from build123d import *
from build123d.topology import SkipClean

# Parameters (mm, degrees)
SKETCH1_W           = 30
SKETCH1_H           = 60
SKETCH1_R           = 1.75
BOSS_EXTRUDE1_DEPTH = 15
SKETCH4_R           = 1.75
BOSS_EXTRUDE3_DEPTH = 30
SKETCH5_W           = 5
SKETCH5_H           = 10
SKETCH5_W_2         = 10
CUT_EXTRUDE1_DEPTH  = 69.738635424
SKETCH6_W           = 7.5
SKETCH6_H           = 15
BOSS_EXTRUDE4_DEPTH = 30
SKETCH7_W           = 30
SKETCH7_H           = 15
BOSS_EXTRUDE5_DEPTH = 10
BOSS_EXTRUDE6_START = 30
SKETCH8_W           = 30
SKETCH8_H           = 15
SKETCH8_R           = 1.75
BOSS_EXTRUDE6_DEPTH = 30


with BuildPart() as part:
    # Sketch1 → Boss-Extrude1 (new body)
    with BuildSketch(Plane.XY):
        with Locations((15, 30)):
            Rectangle(SKETCH1_W, SKETCH1_H)
        with Locations((15, 10)):
            Circle(SKETCH1_R, mode=Mode.SUBTRACT)
    extrude(amount=BOSS_EXTRUDE1_DEPTH)

    # Sketch4 → Boss-Extrude3 (add)
    with BuildSketch(Plane(origin=(30, 0, 0), x_dir=(0, 0, -1), z_dir=(1, 0, 0))):
        with BuildLine():
            Line((-15, 15), (-20, 15))
            ThreePointArc((-20, 15), (-25, 20), (-20, 25))
            Line((-20, 25), (-15, 25))
            Line((-15, 25), (-15, 15))
        make_face()
        with Locations((-20, 20)):
            Circle(SKETCH4_R, mode=Mode.SUBTRACT)
    extrude(amount=-BOSS_EXTRUDE3_DEPTH)

    # Sketch5 → Cut-Extrude1 (cut, through all)
    with BuildSketch(Plane.XY.offset(15)):
        with Locations((2.5, 20)):
            Rectangle(SKETCH5_W, SKETCH5_H)
        with Locations((15, 20)):
            Rectangle(SKETCH5_W_2, SKETCH5_H)
        with Locations((27.5, 20)):
            Rectangle(SKETCH5_W, SKETCH5_H)
    extrude(amount=CUT_EXTRUDE1_DEPTH, mode=Mode.SUBTRACT)

    # Sketch6 → Boss-Extrude4 (add)
    with BuildSketch(Plane.XY.offset(15)):
        with Locations((3.75, 7.5)):
            Rectangle(SKETCH6_W, SKETCH6_H)
        with Locations((26.25, 7.5)):
            Rectangle(SKETCH6_W, SKETCH6_H)
    extrude(amount=BOSS_EXTRUDE4_DEPTH)

    # Sketch7 → Boss-Extrude5 (add)
    with BuildSketch(Plane.XY.offset(45)):
        with Locations((15, 7.5)):
            Rectangle(SKETCH7_W, SKETCH7_H)
    extrude(amount=BOSS_EXTRUDE5_DEPTH)

    # Sketch8 → Boss-Extrude6 (add)
    with SkipClean():  # the faces are left unmerged after this step: merging them gives an invalid solid
        with BuildSketch(Plane(origin=(0, 0, 0), x_dir=(-1, 0, 0), z_dir=(0, 0, -1)).offset(BOSS_EXTRUDE6_START)):
            with Locations((-15, 7.5)):
                Rectangle(SKETCH8_W, SKETCH8_H)
            with Locations((-15, 10)):
                Circle(SKETCH8_R, mode=Mode.SUBTRACT)
        extrude(amount=-BOSS_EXTRUDE6_DEPTH)


solid = part.part
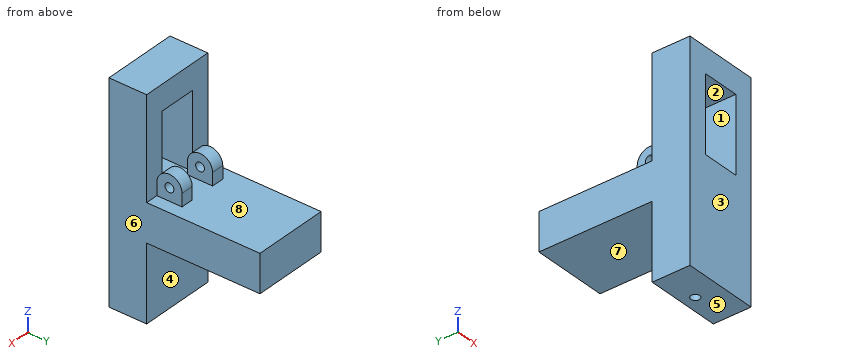
Geometry: final body of the model. Coordinates: model frame, mm. Face numbers are marked on the shaded views. A direction names the side the tool comes from. Give positions to 0.01 mm unless a question says otherwise; leave off trailing zeros. Order: outer loops, then holes, each group sorted by start corner. A loop starts at its lowest first (then second) coordinate and runs counter-clockwise, first axis right, second up. Notation, with made-up numbers: (-16.5, 33) -> (40.5, 33) arc R21 cw to (40.5, 40) -> close; hole circle Ø4 at (-15, -32). An arc over 180 degrees is marked (long way). Answer as a JSON object with one key per item and string values.
Q1. Section D-D (z = 28). Output: boundary loops of the cut face in (x, y), plus the area to 3 significant figures.
Entries:
{"outline": "(0, 0) -> (7.5, 0) -> (7.5, 15) -> (0, 15) -> close; (22.5, 0) -> (30, 0) -> (30, 15) -> (22.5, 15) -> close", "area": "225 mm^2"}
Q2. First-contact query: pin 1 (4 mm diameter, centred on x = 15, y = 10, fed in from -Z); pin 2 (9 mm diameter, centred on x = 15, y = 26, fed in from +Z); pin 3 (6 mm diameter, centred on x = 27, y = 23.5, fed in from -Z); pin 4 (8 mm diameter, centred on y = 22, z = 22, fed in from +X). Flat tips, straight axial feed; report the tip coordinate or a pass-through.
Entries:
{"pin 1": "stops at z = -30", "pin 2": "stops at z = 15", "pin 3": "stops at z = 0", "pin 4": "stops at x = 25"}
Q3. Section B-B (y = 13.5). Output: boundary loops of the cut face in (x, z), plus the area to 3 significant figures.
Entries:
{"outline": "(0, -30) -> (30, -30) -> (30, 55) -> (0, 55) -> close; hole (7.5, 15) -> (22.5, 15) -> (22.5, 45) -> (7.5, 45) -> close", "area": "2,100 mm^2"}
Q4. Access query for the marked faces 1, 2, 3, 4 and 5. Directions: +Z, -Z, +X, -X, +Y, -Y. A direction counts if a zero-diameter tool reaches every point of the face in a straight line with its end or side. Return the directions, or none.
Entries:
{"face 1": "-Y", "face 2": "+Y, -Y", "face 3": "+Z, -Z, +X, -X, -Y", "face 4": "-Z, +X, -X, +Y", "face 5": "-Z, +X, -X, +Y, -Y"}
Q5. Draft query along X for the marked faces 6, 7 and 8. Return one class per face: released by +X, released by -X, zero draft, split by the parting line, or undercut.
Entries:
{"face 6": "released by +X", "face 7": "zero draft", "face 8": "undercut"}
Q6. Section C-C (x = 23.75). Output: boundary loops of the cut face in (y, z).
Entries:
{"outline": "(0, -30) -> (15, -30) -> (15, 0) -> (60, 0) -> (60, 15) -> (25, 15) -> (25, 20) arc R5 ccw to (15, 20) -> (15, 55) -> (0, 55) -> close; hole circle Ø3.5 at (20, 20)"}
Q7. Material intervals for probe 1 along Z at (x, y) = (11.5, 13.5); probe 2 along Y at (x, z) = (8.15, 20); probe 3 along X at (y, z) = (10, 7), sorted ascending.
Entries:
{"probe 1": "z = -30 to 15, 45 to 55", "probe 2": "y = 15 to 18.25, 21.75 to 25", "probe 3": "x = 0 to 13.25, 16.75 to 30"}
Q8. Section A-A (x = 18.5). Output: boundary loops of the cut face in (y, z).
Entries:
{"outline": "(0, -30) -> (15, -30) -> (15, 0) -> (60, 0) -> (60, 15) -> (0, 15) -> close; (0, 45) -> (15, 45) -> (15, 55) -> (0, 55) -> close"}
